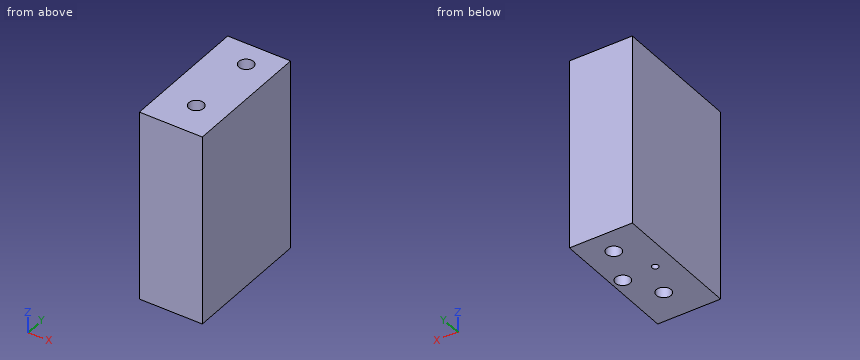
```python
from build123d import *

# Parameters (mm, degrees)
F0_W      = 99.9017828144
F0_H      = 47.2273882478
F1_DEPTH  = 152.4
F2_DEPTH  = 50.8
F3_DEPTH  = 50.8
F4_DEPTH  = 50.8
F5_DEPTH  = 50.8
F7_D      = 11.50874
F10_D     = 11.50874
F10_DEPTH = 76.2
F10_TIP   = 3.4575743203
F11_D     = 5.1054
F11_DEPTH = 76.2
F11_TIP   = 1.5338169022


with BuildPart() as f1:
    # F0 (on Front) → F1 (new body)
    with BuildSketch(Plane.XZ):
        with Locations((43.5557949822, 16.1829041317)):
            Rectangle(F0_W, F0_H)
    extrude(amount=F1_DEPTH)

    # F2 (add): a face of the model
    f2_faces = [f1.faces().sort_by_distance(p)[0] for p in [
        (43.5557949822, -76.2, 39.7965982556),
    ]]
    extrude(f2_faces, amount=F2_DEPTH)

    # F3 (add): a face of the model
    f3_faces = [f1.faces().sort_by_distance(p)[0] for p in [
        (43.5557949822, -76.2, 90.5965982556),
    ]]
    extrude(f3_faces, amount=F3_DEPTH)

    # F4 (cut): a face of the model
    f4_faces = [f1.faces().sort_by_distance(p)[0] for p in [
        (-6.395096425, -76.2, 66.9829041317),
    ]]
    extrude(f4_faces, amount=-F4_DEPTH, mode=Mode.SUBTRACT)

    # F5 (cut): a face of the model
    f5_faces = [f1.faces().sort_by_distance(p)[0] for p in [
        (68.9557949822, 0, 66.9829041317),
    ]]
    extrude(f5_faces, amount=-F5_DEPTH, mode=Mode.SUBTRACT)

    # F7 (through all)
    with Locations(Plane(origin=(0, 0, -7.4307899922), x_dir=(1, 0, 0), z_dir=(0, 0, -1))):
        with Locations((70.703163743, 125.7567703724), (71.8431398273, 70.0071305037)):
            Hole(F7_D / 2)

    # F10
    with Locations(Plane(origin=(0, 0, -7.4307899922), x_dir=(1, 0, 0), z_dir=(0, 0, -1))):
        with Locations((85.044786334, 99.7990220785)):
            Hole(F10_D / 2, depth=F10_DEPTH)
            with Locations((0, 0, -(F10_DEPTH + F10_TIP / 2))):  # 118° drill point
                Cone(0, F10_D / 2, F10_TIP, mode=Mode.SUBTRACT)

    # F11
    with Locations(Plane(origin=(0, 0, -7.4307899922), x_dir=(1, 0, 0), z_dir=(0, 0, -1))):
        with Locations((59.2490546405, 99.0386679769)):
            Hole(F11_D / 2, depth=F11_DEPTH)
            with Locations((0, 0, -(F11_DEPTH + F11_TIP / 2))):  # 118° drill point
                Cone(0, F11_D / 2, F11_TIP, mode=Mode.SUBTRACT)


solid = f1.part
```
Model file for the job. Use its own axes, mm. Give positions to 0.01 mm unless a question says otherwise; leave off trailing zeros. Loops run counter-clockwise (first coordinate to the right, second up) from the corner with the lowest first, then second, coordinate; pieces in that order, holes last. Notation, with made-up numbers: M 74,-30.5 L 86,-30.5 A29 cw 86,-6.5 Z; hole C 1,83 d1. An arc over 180 degrees is marked long. Use one line per item in the form item = value.
Item 1: Slice it at B-B on y = -129.5. List the corners of the cut face in (x, z).
Filled in:
outline = M 44.4,-7.43 L 66.33,-7.43 L 66.33,141.4 L 44.4,141.4 Z; M 75.07,-7.43 L 93.51,-7.43 L 93.51,141.4 L 75.07,141.4 Z
Item 2: Flat gauge pin, fed straight in: pin 1 Ø4.5 at (x, y) = (59.25, -99.04) entering from -Z. Where does the tip first touch, or does it go through?
Filled in:
pin_1 = 68.95
Item 3: Drill centre lines: L1, parallel to Y at x = 75.5, z = 8; L2, parallel to Y at x = 67.5, z = 83; L3, parallel to X at y = -131, z = 36. Where is each one in solid material? Low to high.
Filled in:
L1 = -152.4 to -128.94, -122.58 to -74.45, -65.56 to -50.8
L2 = -152.4 to -130.54, -120.98 to -73.78, -66.23 to -50.8
L3 = 44.4 to 68.33, 73.07 to 93.51
Item 4: Slice it at A-A on x = 71. List the corners of the cut face in (y, z).
Filled in:
outline = M -152.4,-7.43 L -131.5,-7.43 L -131.5,141.4 L -152.4,141.4 Z; M -120.01,-7.43 L -75.7,-7.43 L -75.7,141.4 L -120.01,141.4 Z; M -64.31,-7.43 L -50.8,-7.43 L -50.8,141.4 L -64.31,141.4 Z
Item 5: Slice it at C-C on z = 85. List the corners of the cut face in (x, y).
Filled in:
outline = M 44.4,-152.4 L 93.51,-152.4 L 93.51,-50.8 L 44.4,-50.8 Z; hole C 70.7,-125.76 d11.51; hole C 71.84,-70.01 d11.51
